CAD build for the part. Positions are in the model's coordinates, mm. Face numbers are marked on the shaded views. A direction names the side the tool comes from. Coordinates: 2 decimals unless noted, no trailing zeros. Loops run counter-clockwise (first coordinate to the right, second up) from the corner with the lowest first, then second, coordinate; pieces in that order, holes last. Notation, with made-up numbers: (-5, 46.25) -> (42, 46.25) arc R20 ccw to (42, 66.25) -> close; hole circle Ø4 at (-15, 18). An arc over 180 degrees is marked (long way). Answer as CSV lines item,"result". Start each with the question number.
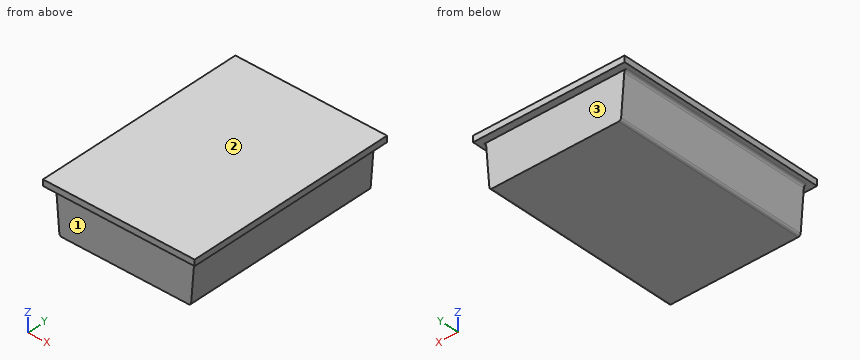
from build123d import *

# Parameters (mm, degrees)
F1_DEPTH = 420
F3_DEPTH = 14


# Not quite as in the source:
# - a pattern or mirror of a feature is missing from the dataset's text; its kind, count and spacing are read off the source's solid


with BuildPart() as f1:
    # F0 (on Front) → F1 (new body)
    with BuildSketch(Plane.XZ):
        with BuildLine():
            Line((150, 0), (0, 0))
            Line((0, 0), (-150, 0))
            Line((-150, 0), (-150, -12))
            Line((-150, -12), (-141.6180664814, -12))
            ThreePointArc((-141.6180664814, -12), (-138.2256023722, -13.3269648425), (-136.633810504, -16.6035250927))
            Line((-136.633810504, -16.6035250927), (-130.366189496, -95.3964749073))
            ThreePointArc((-130.366189496, -95.3964749073), (-128.7743976278, -98.6730351575), (-125.3819335186, -100))
            Line((-125.3819335186, -100), (0, -100))
            Line((0, -100), (125.3819335186, -100))
            ThreePointArc((125.3819335186, -100), (128.7743976278, -98.6730351575), (130.366189496, -95.3964749073))
            Line((130.366189496, -95.3964749073), (136.633810504, -16.6035250927))
            ThreePointArc((136.633810504, -16.6035250927), (138.2256023722, -13.3269648425), (141.6180664814, -12))
            Line((141.6180664814, -12), (150, -12))
            Line((150, -12), (150, 0))
        make_face()
    extrude(amount=F1_DEPTH)

    # F2 (on face) → F3 (cut)
    with BuildSketch(Plane.XZ.offset(420)):
        with BuildLine():
            Line((141.6180664814, -12), (-141.6180664814, -12))
            ThreePointArc((-141.6180664814, -12), (-138.2256023722, -13.3269648425), (-136.633810504, -16.6035250927))
            Line((-136.633810504, -16.6035250927), (-130.366189496, -95.3964749073))
            ThreePointArc((-130.366189496, -95.3964749073), (-128.7743976278, -98.6730351575), (-125.3819335186, -100))
            Line((-125.3819335186, -100), (125.3819335186, -100))
            ThreePointArc((125.3819335186, -100), (128.7743976278, -98.6730351575), (130.366189496, -95.3964749073))
            Line((130.366189496, -95.3964749073), (136.633810504, -16.6035250927))
            ThreePointArc((136.633810504, -16.6035250927), (138.2256023722, -13.3269648425), (141.6180664814, -12))
        make_face()
    f3 = extrude(amount=-F3_DEPTH, mode=Mode.SUBTRACT)

    # F3_copies: F3 across plane
    add(f3.mirror(Plane.ZX.offset(-210)), mode=Mode.SUBTRACT)


solid = f1.part
Item 1: Saw through at D-D (z = -88.5). Write the cut outline in (x, y).
Item 2: Saw through at C-C (z = -50.5). Write the cut outline in (x, y), plus the area to 3 significant figures.
Item 3: Which spindle directions (+Z, -Z, +X, -X, +Y, -Y) get a long thin tool onto all of the face, cutting with end or side? Do the marked faces 1, 2 and 3. Say none if no direction does.
Item 4: Saw through at B-B (x = -8). Write the cut outline in (y, z), plus the area to 3 significant figures.
Item 5: Wall check: probe 1 along Y at (x, z) = (74, -56.5); probe 2 along X at (y, z) = (-283, -51.5); probe 3 along X at (y, z) = (-281.5, -24). Give the ranges that are in metal, low to high.
Item 6: Flat gauge pins, fed straight in: pin 1 Ø5 at (y, z) = (-373, -45.5) entering from +X; pin 2 Ø8 at (y, z) = (-45.5, -42) entering from +X; pin 3 Ø4 at (y, z) = (-332, -17.5) entering from -X. Where does each tip first touch, or does it go through?
Item 7: Saw through at A-A (y = -87.5). Write the cut outline in (x, z).
Geometry check:
1,outline,"(-130.91, -406) -> (130.91, -406) -> (130.91, -14) -> (-130.91, -14) -> close"
2,outline,"(-133.94, -406) -> (133.94, -406) -> (133.94, -14) -> (-133.94, -14) -> close"
2,area,"105,000 mm2"
3,face 1,"-Z, +X, -X, -Y"
3,face 2,"+Z, +X, -X, +Y, -Y"
3,face 3,"-Z, +X, -X, +Y"
4,outline,"(-420, -12) -> (-406, -12) -> (-406, -100) -> (-14, -100) -> (-14, -12) -> (0, -12) -> (0, 0) -> (-420, 0) -> close"
4,area,"39,500 mm2"
5,probe 1,"-406 to -14"
5,probe 2,"-133.86 to 133.86"
5,probe 3,"-136.05 to 136.05"
6,pin 1,"x = 134.53"
6,pin 2,"x = 134.93"
6,pin 3,"x = -136.85"
7,outline,"(-150, -12) -> (-141.62, -12) arc R5 cw to (-136.63, -16.6) -> (-130.37, -95.4) arc R5 ccw to (-125.38, -100) -> (125.38, -100) arc R5 ccw to (130.37, -95.4) -> (136.63, -16.6) arc R5 cw to (141.62, -12) -> (150, -12) -> (150, 0) -> (-150, 0) -> close"
